Can you work these out from the model? Positions are in its coordinate system, mm. Face numbers are marked on the shaded views. A direction names the side the tool comes from. Give positions to 0.01 mm unless a question says otherwise; leave off trailing zeros. Write each loop counter-clockwise with the first axis right and the second up, starting at its lowest first coordinate (ties: lowest second). Pieces come first, ordered by that corner, then holes. Notation, with made-up numbers: (1, 54.5) - (40, 54.5) arc R28 cw to (40, 82.5) - close; hole circle Ø4 at (-24, 53). An arc over 180 degrees is marked (long way). Return JSON: item names as keys, results as strings. Group by question number.
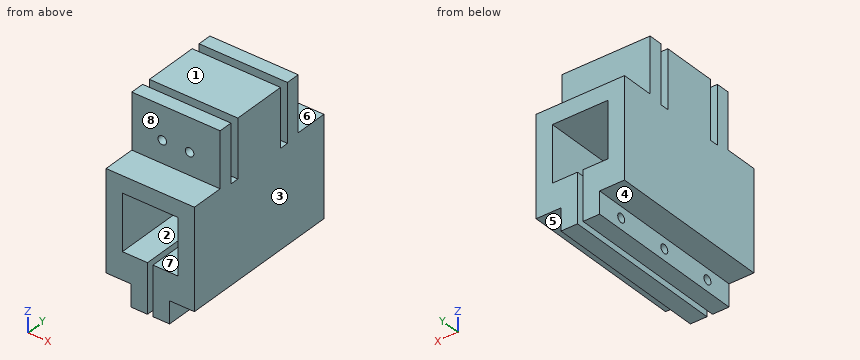
Autodesk Inventor part; units mm, degrees
ref_plane "YZ Plane" through (0, 0, 0) normal (1, 0, 0) x (0, 1, 0)
ref_plane "XZ Plane" through (0, 0, 0) normal (0, 1, 0) x (-1, 0, 0)
ref_plane "XY Plane" through (0, 0, 0) normal (0, 0, 1) x (1, 0, 0)
sketch "Sketch1" plane through (0, 0, 0) normal (0, 0, 1) x (1, 0, 0)
  line L0 (0, 0) -> (32, 0)
  line L1 (32, 0) -> (32, 60)
  line L2 (32, 60) -> (0, 60)
  line L3 (0, 60) -> (0, 0)
  dimension "d0" = 32
  dimension "d1" = 60
extrude "Extrusion1" add sketch "Sketch1" along normal blind 6
sketch "Sketch3" plane through (0, 0, 6) normal (0, 0, 1) x (1, 0, 0)
  line L0 (32, 0) -> (32, 60)
  line L1 (32, 60) -> (0, 60)
  line L2 (0, 60) -> (0, 0)
  line L3 (0, 0) -> (32, 0)
  line L4 (0, 30) -> (32, 30) construction
  line L5 (32, 0) -> (32, 60) construction
  line L6 (0, 60) -> (0, 0)
  line L7 (0, 39.9) -> (32, 39.9)
  line L8 (32, 39.9) -> (32, 20.1)
  line L9 (32, 20.1) -> (0, 20.1)
  line L10 (0, 20.1) -> (0, 39.9)
  line L11 (0, 43.1) -> (32, 43.1)
  line L12 (32, 43.1) -> (32, 48.1)
  line L13 (32, 48.1) -> (0, 48.1)
  line L14 (0, 48.1) -> (0, 43.1)
  line L15 (0, 16.9) -> (32, 16.9)
  line L16 (32, 16.9) -> (32, 11.9)
  line L17 (32, 11.9) -> (0, 11.9)
  line L18 (0, 11.9) -> (0, 16.9)
  point P0 (0, 11.9)
  point P1 (0, 20.1)
  point P2 (0, 48.1)
  point P3 (0, 43.1)
  dimension "d6" = 30
  dimension "d7" = 60
  dimension "d8" = 9.9
  dimension "d9" = 9.9
  dimension "d10" = 5
  dimension "d11" = 3.2
  dimension "d12" = 3.2
  dimension "d13" = 5
extrude "Extrusion2" add sketch "Sketch3" along normal blind 20 contours L17 L2 L15 L0 | L9 L2 L7 L0 | L11 L2 L13 L0
sketch "Sketch4" plane through (0, 48.1, 6) normal (0, 1, 0) x (1, 0, 0)
  line L0 (0, 0) -> (32, 0)
  line L1 (0, 0) -> (0, -20)
  line L2 (32, -20) -> (0, -20)
  line L3 (32, 0) -> (32, -20)
  circle A0 centre (11.05, -8) radius 1.55
  circle A1 centre (20.95, -8) radius 1.55
  line L4 (0, -20) -> (32, -20) construction
  line L5 (16, -20) -> (16, 0) construction
  point P0 (0, 6)
  dimension "d16" = 3.1
  dimension "d17" = 3.1
  dimension "d18" = 4.95
  dimension "d19" = 4.95
  dimension "d20" = 8
  dimension "d21" = 8
extrude "Extrusion3" cut sketch "Sketch4" against normal blind 100 contours A0 | A1
ref_plane "Work Plane1" through (16, 0, 0) normal (1, 0, 0) x (0, 0, -1)
ref_plane "Work Plane3" through (0, 30, 6) normal (0, 1, 0) x (1, 0, 0)
sketch "Sketch14" plane through (0, 60, 0) normal (0, 1, 0) x (1, 0, 0)
  line L0 (32, 0) -> (0, 0)
  line L1 (5.9, 0) -> (26.1, 0)
  line L2 (26.1, 0) -> (26.1, 20.2)
  line L3 (26.1, 20.2) -> (5.9, 20.2)
  line L4 (5.9, 20.2) -> (5.9, 0)
  line L5 (0, 0) -> (32, 0)
  line L6 (32, 0) -> (32, 30)
  line L7 (32, 30) -> (0, 30)
  line L8 (0, 30) -> (0, 0)
  line L9 (32, 0) -> (32, -6)
  line L10 (9, 20.2) -> (15, 20.2)
  line L11 (15, 20.2) -> (15, 38)
  line L12 (15, 38) -> (9, 38)
  line L13 (9, 38) -> (9, 20.2)
  line L14 (23, 20.2) -> (17, 20.2)
  line L15 (17, 20.2) -> (17, 38)
  line L16 (17, 38) -> (23, 38)
  line L17 (23, 38) -> (23, 20.2)
  line L18 (16, 46) -> (16, -38)
  point P0 (23, 30)
  point P1 (9, 30)
  dimension "d74" = 20.2
  dimension "d75" = 20.2
  dimension "d76" = 30
  dimension "d77" = 5.9
  dimension "d78" = 32
  dimension "d79" = 1
  dimension "d80" = 1
  dimension "d81" = 6
  dimension "d82" = 6
  dimension "d83" = 8
  dimension "d85" = 8
extrude "Extrusion12" add sketch "Sketch14" against normal blind 60 contours L0 L2 L3 L17 L7 L6 | L17 L3 L15 L7 | L7 L15 L16 L17 | L0 L8 L7 L13 L3 L4 | L3 L13 L7 L11 | L7 L13 L12 L11
sketch "Sketch15" plane through (23, 60, -30) normal (1, 0, 0) x (0, 0, -1)
  circle A0 centre (4, -10) radius 1.6
  circle A1 centre (4, -30) radius 1.6
  circle A2 centre (4, -50) radius 1.6
  line L0 (8, -60) -> (0, -60)
  line L1 (0, 0) -> (8, 0)
  line L2 (8, 0) -> (8, -60)
  point P0 (-30, -60)
  dimension "d88" = 3.2
  dimension "d89" = 3.2
  dimension "d90" = 3.2
  dimension "d91" = 10
  dimension "d92" = 10
  dimension "d93" = 30
  dimension "d94" = 4
extrude "Extrusion13" cut sketch "Sketch15" against normal blind 60
sketch "Sketch16" plane through (0, 0, 6) normal (0, 0, 1) x (1, 0, 0)
  line L0 (0, 39.9) -> (32, 39.9)
  line L1 (32, 39.9) -> (32, 43.1)
  line L2 (32, 43.1) -> (0, 43.1)
  line L3 (0, 43.1) -> (0, 39.9)
  line L4 (0, 16.9) -> (32, 16.9)
  line L5 (32, 16.9) -> (32, 20.1)
  line L6 (32, 20.1) -> (0, 20.1)
  line L7 (0, 20.1) -> (0, 16.9)
  point P0 (0, 0)
extrude "Extrusion14" cut sketch "Sketch16" against normal blind 1
equation "\"d6\" = 0.5 * d7"
equation "\"d77\" = -0.5 * d74 + 0.5 * d78"
properties part number "Drone_mount"
1) Will these pins go through, and if not, where does the flat tip stop? pin 1 Ø10.5 at (x, z) = (22, 15) entering from +Y; pin 2 Ø3.5 at (y, z) = (10, -34) entering from +X; pin 3 Ø10.5 at (x, z) = (15.5, 11.5) entering from -Y.
2) Imagine slicing it at A-A, the plane y = 50. Write out the boundary of the cut face in (x, z).
3) On a 3-axis mill with a long thin cutter (end or side, diameter ignored), from which of +Z, -Z, +X, -X, +Y, -Y can I reach the whole of each face in a straight line? I mean the marked faces 4, 5, 6, 7 and 8. Say none if no direction works.
4) Imagine slicing it at C-C, the plane y = 30. Write out the boundary of the cut face in (x, z), and give its area (3 significant figures).
5) We'd pull the mould along X, two halves only. Please class the marked faces 1, 2 and 3: pulls with the +X half, pulls with the -X half, needs draft (parallel to the pull), parting line crosses it, or undercut.
6) Imagine slicing it at D-D, the plane x = 8. Write out the boundary of the cut face in (y, z).
7) I need wall thicknesses on line 1 along Y through (x, z) = (1, 23); line 2 along Y through (x, z) = (20.5, -34); line 3 along Z through (x, y) = (21, 25). Which ranges of each line are inside material? Lowest first, please.
8) Imagine slicing it at B-B, the plane z = -21. Write out the boundary of the cut face in (x, y).
Resolved:
{
 "1": {"pin 1": "y = 48.1", "pin 2": "x = 23", "pin 3": "y = 11.9"},
 "2": {"outline": "(0, -30) - (9, -30) - (9, -32.4) - (15, -32.4) - (15, -20.2) - (5.9, -20.2) - (5.9, 0) - (26.1, 0) - (26.1, -20.2) - (17, -20.2) - (17, -32.4) - (23, -32.4) - (23, -30) - (32, -30) - (32, 6) - (0, 6) - close; (9, -38) - (15, -38) - (15, -35.6) - (9, -35.6) - close; (17, -38) - (23, -38) - (23, -35.6) - (17, -35.6) - close"},
 "3": {"face 4": "-Z, -X, +Y, -Y", "face 5": "-Z, +X, +Y, -Y", "face 6": "+Z, +X, -X, +Y", "face 7": "+Y, -Y", "face 8": "+Z, +X, -X, -Y"},
 "4": {"outline": "(0, -30) - (9, -30) - (9, -32.4) - (15, -32.4) - (15, -20.2) - (5.9, -20.2) - (5.9, 0) - (26.1, 0) - (26.1, -20.2) - (17, -20.2) - (17, -32.4) - (23, -32.4) - (23, -30) - (32, -30) - (32, 26) - (0, 26) - close; (9, -38) - (15, -38) - (15, -35.6) - (9, -35.6) - close; (17, -38) - (23, -38) - (23, -35.6) - (17, -35.6) - close; hole circle Ø3.1 at (11.05, 14); hole circle Ø3.1 at (20.95, 14)", "area": "1,410 mm^2"},
 "5": {"face 1": "needs draft", "face 2": "undercut", "face 3": "pulls with the +X half"},
 "6": {"outline": "(0, -30) - (60, -30) - (60, -20.2) - (0, -20.2) - close; (0, 0) - (60, 0) - (60, 6) - (48.1, 6) - (48.1, 26) - (43.1, 26) - (43.1, 5) - (39.9, 5) - (39.9, 26) - (20.1, 26) - (20.1, 5) - (16.9, 5) - (16.9, 26) - (11.9, 26) - (11.9, 6) - (0, 6) - close"},
 "7": {"line 1": "11.9 to 16.9, 20.1 to 39.9, 43.1 to 48.1", "line 2": "0 to 8.4, 11.6 to 28.4, 31.6 to 48.4, 51.6 to 60", "line 3": "-38 to -20.2, 0 to 12.45, 15.55 to 26"},
 "8": {"outline": "(0, 0) - (15, 0) - (15, 60) - (0, 60) - close; (17, 0) - (32, 0) - (32, 60) - (17, 60) - close"}
}
